Could you check a few things on this model? Use its own coordinates, in mm. A direction names the side the tool comes from. Coordinates: 2 decimals unless noted, no trailing zeros. Order: outer loops, then holes, each group sorted by start corner. A loop starts at its lowest first (then second) coordinate and runs counter-clockwise, first axis right, second up. Notation, with made-up numbers: (71, -37) -> (93, -37) arc R30 ccw to (93, 2) -> close; hole circle Ø1 at (7, -10.5). An arc over 180 degrees is marked (long way). Use a Markdown table: item, result. Add a question column.
1) If we section it at B-B (x = 0): Write out the boundary of the cut face in (y, z).
2) If we section it at A-A (z = 0.85): Write out the boundary of the cut face in (x, y).
3) If we section it at D-D (x = -6): Write out the boundary of the cut face in (y, z).
4) If we section it at C-C (y = -11.25): Write out the boundary of the cut face in (x, z), plus the area to 3 significant figures.
5) Will these pins go through, and if not, where does the flat tip stop? pin 1 Ø1.1 at (y, z) = (6.5, 1.5) entering from -X; pin 2 Ø1 at (y, z) = (10, 1.5) entering from +X; pin 3 Ø0.6 at (x, z) = (7, 1) entering from -Y.
6) Thinking about a two-plate mould opening in Y: for faces 4 (the cylindrical face through (7.465, 16.449, 1.085)), 5 (the cylindrical face through (-0.255, -12.714, 1.085)), 6 (the cylindrical face through (-5.26, -16.45, 1.08)), which applies, +Y half, -Y half, draft (parallel to the pull), parting line (faces both ways), or undercut?
7) If I drill on L1, parallel to X at y = -10.5, z = 0.55; L2, parallel to X at y = -14.5, z = 1.65; L3, parallel to X at y = 7, z = 2.05, over which ranges is the centre line in solid material (lowest first)? Write a range as [from, to].
8) Which directions (+Z, -Z, +X, -X, +Y, -Y) give clear straight access to the entire face, cutting with the end or side of a thin tool? Please do faces 1 (the flat face through (0, 16.75, 1)), 2 (the flat face through (7, 11.25, 1)), 3 (the flat face through (1.57, 6, 1)).
```python
from build123d import *

# Parameters (mm, degrees)
SKETCH1_R           = 1.5
BOSS_EXTRUDE1_DEPTH = 2.2


with BuildPart() as part:
    # Sketch1 → Boss-Extrude1 (new body)
    with BuildSketch(Plane.XY):
        with BuildLine():
            Line((-4.547445363, -16.75), (4.756345477, -16.75))
            ThreePointArc((4.756345477, -16.75), (5.463452258, -16.457106781), (5.756345477, -15.75))
            Line((5.756345477, -15.75), (5.756345477, 11.25))
            Line((5.756345477, 11.25), (7.75, 11.25))
            Line((7.75, 11.25), (7.75, 15.75))
            ThreePointArc((7.75, 15.75), (7.457106781, 16.457106781), (6.75, 16.75))
            Line((6.75, 16.75), (-6.75, 16.75))
            ThreePointArc((-6.75, 16.75), (-7.457106781, 16.457106781), (-7.75, 15.75))
            Line((-7.75, 15.75), (-7.75, 11.213631532))
            Line((-7.75, 11.213631532), (-5.65, 11.25))
            Line((-5.65, 11.25), (-5.547438151, -15.753798025))
            ThreePointArc((-5.547438151, -15.753798025), (-5.253208062, -16.458448313), (-4.547445363, -16.75))
        make_face()
        with Locations((0.070153023, -11.25)):
            Circle(SKETCH1_R, mode=Mode.SUBTRACT)
        with BuildLine():
            Line((-1.429846977, 5.35), (-1.429846977, 7.55))
            ThreePointArc((-1.429846977, 7.55), (0.070153023, 9.05), (1.570153023, 7.55))
            Line((1.570153023, 7.55), (1.570153023, 5.35))
            ThreePointArc((1.570153023, 5.35), (0.070153023, 3.85), (-1.429846977, 5.35))
        make_face(mode=Mode.SUBTRACT)
    extrude(amount=BOSS_EXTRUDE1_DEPTH)


solid = part.part
```
Answer sheet:
| question | item | result |
|---|---|---|
| 1 | outline | (-16.75, 0) -> (-12.75, 0) -> (-12.75, 2.2) -> (-16.75, 2.2) -> close; (-9.75, 0) -> (3.85, 0) -> (3.85, 2.2) -> (-9.75, 2.2) -> close; (9.05, 0) -> (16.75, 0) -> (16.75, 2.2) -> (9.05, 2.2) -> close |
| 2 | outline | (-7.75, 11.21) -> (-5.65, 11.25) -> (-5.55, -15.75) arc R1 ccw to (-4.55, -16.75) -> (4.76, -16.75) arc R1 ccw to (5.76, -15.75) -> (5.76, 11.25) -> (7.75, 11.25) -> (7.75, 15.75) arc R1 ccw to (6.75, 16.75) -> (-6.75, 16.75) arc R1 ccw to (-7.75, 15.75) -> close; hole circle Ø3 at (0.07, -11.25); hole (-1.43, 5.35) arc R1.5 ccw to (1.57, 5.35) -> (1.57, 7.55) arc R1.5 ccw to (-1.43, 7.55) -> close |
| 3 | outline | (11.24, 0) -> (16.75, 0) -> (16.75, 2.2) -> (11.24, 2.2) -> close |
| 4 | outline | (-5.56, 0) -> (-1.43, 0) -> (-1.43, 2.2) -> (-5.56, 2.2) -> close; (1.57, 0) -> (5.76, 0) -> (5.76, 2.2) -> (1.57, 2.2) -> close |
| 4 | area | 18.3 mm2 |
| 5 | pin 1 | x = -5.63 |
| 5 | pin 2 | x = 5.76 |
| 5 | pin 3 | y = 11.25 |
| 6 | face 4 | +Y half |
| 6 | face 5 | undercut |
| 6 | face 6 | -Y half |
| 7 | L1 | [-5.57, -1.23], [1.37, 5.76] |
| 7 | L2 | [-5.55, 5.76] |
| 7 | L3 | [-5.63, -1.43], [1.57, 5.76] |
| 8 | face 1 | +Z, -Z, +X, -X, +Y |
| 8 | face 2 | +Z, -Z, +X, -Y |
| 8 | face 3 | +Z, -Z |
